```python
from build123d import *

# Parameters (mm, degrees)
ESQUISSE1_R                  = 32
BOSS_EXTRU_1_DEPTH           = 15
ESQUISSE2_R                  = 36
ESQUISSE2_R_2                = 32
BOSS_EXTRU_2_DEPTH           = 8
CHANFREIN1_SIZE              = 1
CONG_1_R                     = 0.2
ESQUISSE3_R                  = 4.25
ENL_V_MAT_EXTRU_1_DEPTH      = 24
ESQUISSE4_R                  = 7
ENL_V_MAT_EXTRU_2_DEPTH      = 8
R_P_TITION_CIRCULAIRE1_COUNT = 3


with BuildPart() as part:
    # Esquisse1 → Boss.-Extru.1 (new body)
    with BuildSketch(Plane.XY):
        with BuildLine():
            Line((-7, 54), (7, 54))
            Line((7, 54), (7, 52))
            ThreePointArc((7, 52), (8.464466094, 48.464466094), (12, 47))
            Line((12, 47), (42, 47))
            Line((42, 47), (42, -11))
            ThreePointArc((42, -11), (43.464466094, -14.535533906), (47, -16))
            Line((47, -16), (50, -16))
            Line((50, -16), (50, -46))
            Line((50, -46), (-50, -46))
            Line((-50, -46), (-50, -16))
            Line((-50, -16), (-47, -16))
            ThreePointArc((-47, -16), (-43.464466094, -14.535533906), (-42, -11))
            Line((-42, -11), (-42, 47))
            Line((-42, 47), (-12, 47))
            ThreePointArc((-12, 47), (-8.464466094, 48.464466094), (-7, 52))
            Line((-7, 52), (-7, 54))
        make_face()
        Circle(ESQUISSE1_R, mode=Mode.SUBTRACT)
    extrude(amount=BOSS_EXTRU_1_DEPTH)

    # Esquisse2 → Boss.-Extru.2 (add)
    with BuildSketch(Plane.XY.offset(15)):
        with Locations(Location((0, 0, 0), (0, 0, 180))):  # turned: the seam where the file's is
            Circle(ESQUISSE2_R)
        Circle(ESQUISSE2_R_2, mode=Mode.SUBTRACT)
    extrude(amount=BOSS_EXTRU_2_DEPTH)

    # Chanfrein1
    chanfrein1_edges = [part.edges().sort_by_distance(p)[0] for p in [
        (36, 0, 23),
    ]]
    chamfer(chanfrein1_edges, length=CHANFREIN1_SIZE)

    # Congé1
    cong_1_edges = [part.edges().sort_by_distance(p)[0] for p in [
        (36, 0, 15),
    ]]
    fillet(cong_1_edges, radius=CONG_1_R)

    # Esquisse3 → Enlèv. mat.-Extru.1 (cut, through all)
    with BuildSketch(Plane(origin=(0, 0, 0), x_dir=(-1, 0, 0), z_dir=(0, 0, -1))):
        with Locations((0, 46)):
            Circle(ESQUISSE3_R)
    enl_v_mat_extru_1 = extrude(amount=-ENL_V_MAT_EXTRU_1_DEPTH, mode=Mode.SUBTRACT)

    # Esquisse4 → Enlèv. mat.-Extru.2 (cut)
    with BuildSketch(Plane(origin=(0, 0, 0), x_dir=(-1, 0, 0), z_dir=(0, 0, -1))):
        with Locations((0, 46)):
            Circle(ESQUISSE4_R)
    enl_v_mat_extru_2 = extrude(amount=-ENL_V_MAT_EXTRU_2_DEPTH, mode=Mode.SUBTRACT)

    # Répétition circulaire1: Enlèv. mat.-Extru.1, Enlèv. mat.-Extru.2 ×3 about axis
    r_p_tition_circulaire1_axis = Axis((0, 0, 0), (0, 0, 1))
    add([enl_v_mat_extru_1.rotate(r_p_tition_circulaire1_axis, i * 360 / R_P_TITION_CIRCULAIRE1_COUNT) for i in range(1, R_P_TITION_CIRCULAIRE1_COUNT)], mode=Mode.SUBTRACT)
    add([enl_v_mat_extru_2.rotate(r_p_tition_circulaire1_axis, i * 360 / R_P_TITION_CIRCULAIRE1_COUNT) for i in range(1, R_P_TITION_CIRCULAIRE1_COUNT)], mode=Mode.SUBTRACT)


solid = part.part
```
Here's how the part is built. I have some questions about the finished solid (model axes, mm). A direction names the side the tool comes from. Coordinates: 2 decimals unless noted, no trailing zeros. Write each loop counter-clockwise with the first axis right and the second up, starting at its lowest first coordinate (ties: lowest second). Pieces come first, ordered by that corner, then holes. Notation, with made-up numbers: (-14.75, 59.5) -> (4.25, 59.5) arc R29 ccw to (4.25, 88.5) -> close; hole circle Ø6 at (9, -28). An arc over 180 degrees is marked (long way). Use a Markdown table: item, result. Add a question column.
(1) Please list where these lines run through material, in increasing order: line 1 (Y direction, x = 0, z = 13); line 2 (Y direction, x = 0, z = 6.25); line 3 (Y direction, x = -23, z = 4).
(2) I'm going to push flat-ended pins straight in: P1, Ø3.5, axis at x = -48.5, z = 7, coming from the +Y side; P2, Ø1, axis at y = 53, z = 11, coming from the +X side; P3, Ø2, axis at y = 53, z = 11, coming from the -X side; P4, Ø5, axis at x = 39.84, y = -23, coming from the +Z side. Where does each tip first touch, or does it pass through?
(3) If we section it at D-D, the plane z = 5.5: Write out the boundary of the cut face in (x, y).
(4) If we section it at B-B, the plane x = 38.5: Write out the boundary of the cut face in (y, z), and give its area (3 significant figures).
(5) For faces 1 (the cylindrical face through (-43.89, -21.72, 11.45)), 2 (the flat face through (27, 47, 7)), 3 (the flat face through (-5, 46, 8)), 4 (the flat face through (-42, 18, 7)), which set-ups out of +Z, -Z, +X, -X, +Y, -Y let a thin tool reach every point of the face, with its end or its side?
(6) If we section it at A-A, the plane y = 0: Write out the boundary of the cut face in (x, z).
(7) We'd pull the mould along Y, two halves only. Please class faces 5 (the flat face through (26.2, -25.4, 15)), 6 (the cylindrical face through (0.91, 52.94, 3.94)), 7 (the cylindrical face through (26.533, -24.331, 18.552)): +Y half, -Y half, draft (parallel to the pull), parting line (faces both ways), or undercut.
(8) If we section it at C-C, the plane x = 0: Write out the boundary of the cut face in (y, z).
Outcome:
| question | item | result |
|---|---|---|
| 1 | line 1 | y = -46 to -32, 32 to 41.75, 50.25 to 54 |
| 1 | line 2 | y = -46 to -32, 32 to 39, 53 to 54 |
| 1 | line 3 | y = -46 to -22.25, 22.25 to 47 |
| 2 | P1 | stops at y = -15.99 |
| 2 | P2 | stops at x = 7 |
| 2 | P3 | stops at x = -7 |
| 2 | P4 | passes through |
| 3 | outline | (-50, -46) -> (50, -46) -> (50, -16) -> (47, -16) arc R5 cw to (42, -11) -> (42, 47) -> (12, 47) arc R5 cw to (7, 52) -> (7, 54) -> (-7, 54) -> (-7, 52) arc R5 cw to (-12, 47) -> (-42, 47) -> (-42, -11) arc R5 cw to (-47, -16) -> (-50, -16) -> close; hole circle Ø14 at (-39.84, -23); hole circle Ø64 at (0, 0); hole circle Ø14 at (0, 46); hole circle Ø14 at (39.84, -23) |
| 4 | outline | (-46, 0) -> (-29.87, 0) -> (-29.87, 8) -> (-27.03, 8) -> (-27.03, 15) -> (-46, 15) -> close; (-18.97, 8) -> (-16.13, 8) -> (-16.13, 0) -> (47, 0) -> (47, 15) -> (-18.97, 15) -> close |
| 4 | area | 1,230 mm^2 |
| 5 | face 1 | +Z, -Z |
| 5 | face 2 | +Z, -Z, +X, +Y |
| 5 | face 3 | -Z |
| 5 | face 4 | +Z, -Z, -X, +Y |
| 6 | outline | (-42, 0) -> (-32, 0) -> (-32, 23) -> (-35, 23) -> (-36, 22) -> (-36, 15.2) arc R0.2 cw to (-36.2, 15) -> (-42, 15) -> close; (32, 0) -> (42, 0) -> (42, 15) -> (36.2, 15) arc R0.2 cw to (36, 15.2) -> (36, 22) -> (35, 23) -> (32, 23) -> close |
| 7 | face 5 | draft |
| 7 | face 6 | undercut |
| 7 | face 7 | parting line |
| 8 | outline | (-46, 0) -> (-32, 0) -> (-32, 23) -> (-35, 23) -> (-36, 22) -> (-36, 15.2) arc R0.2 cw to (-36.2, 15) -> (-46, 15) -> close; (32, 0) -> (39, 0) -> (39, 8) -> (41.75, 8) -> (41.75, 15) -> (36.2, 15) arc R0.2 cw to (36, 15.2) -> (36, 22) -> (35, 23) -> (32, 23) -> close; (50.25, 8) -> (53, 8) -> (53, 0) -> (54, 0) -> (54, 15) -> (50.25, 15) -> close |
